Verification items for the finished model (mm, model axes). Face numbers are marked on the shaded views. A direction names the side the tool comes from. Give positions to 0.01 mm unless a question says otherwise; leave off trailing zeros. Loops run counter-clockwise (first coordinate to the right, second up) from the corner with the lowest first, then second, coordinate; pieces in that order, holes last. Notation, with made-up numbers: (-31, 25.25) - (22, 25.25) arc R23 ccw to (22, 51.25) - close; hole circle Ø10 at (55, -9.5). An arc over 180 degrees is marked (long way). One line per question, with ' | ' between items. Start each with the question number.
1. Depth check by flat-ended pin: pin 1 Ø10 at (x, z) = (83.5, -2) entering from +Y; pin 2 Ø16 at (x, y) = (82.5, 2.5) entering from -Z; pin 3 Ø10 at (x, y) = (85.5, 2.5) entering from +Z. Enter the tip coordinate at first touch or a pass-through.
2. Thickness scan on line 1 along X through (y, z) = (-10, 9); line 2 along X through (y, z) = (-11, 1); line 3 along Y through (x, z) = (58.5, 5.5). Record the ranges inside material, lowest first. Write a range as from..to.
3. Tool access check on the marked faces 1, 2, 3 and 4. Record the directions out of +Z, -Z, +X, -X, +Y, -Y that give a thin tool (end or side, any length) a straight path to the whole face; none if there is none.
4. Section check A-A, the plane z = -7.75. Enter the section's corners in (x, y), then the cut area to 3 significant figures.
5. Section check B-B, the plane x = 0. Enter the section's corners in (y, z).
6. Section check C-C, the plane z = 1. Enter the section's corners in (x, y).
7. Mould release check, pull along X, two halves, no side actions. Record for the marked faces 5 and 6: +X half, -X half, draft (parallel to the pull), parting line (faces both ways), or undercut.
8. Section check D-D, the plane y = -14. Enter the section's corners in (x, z), then the cut area to 3 significant figures.
Autodesk Fusion 360 part; units mm, degrees
sketch "Sketch1" plane through (0, 0, 0) normal (0, 0, 1) x (1, 0, 0)
  circle A0 centre (0, 0) radius 30
  circle A1 centre (129, 0) radius 20
  line L0 (0, 0) -> (0, 0)
  line L1 (0, 0) -> (0, 0)
  line L2 (0, 0) -> (0, 0)
  line L3 (0, 0) -> (0, 0)
  line L4 (0, 0) -> (0, 0)
  line L5 (0, 0) -> (0, 0)
  line L6 (-11.547, 20) -> (-23.094, 0)
  line L7 (-23.094, 0) -> (-11.547, -20)
  line L8 (-11.547, -20) -> (11.547, -20)
  line L9 (11.547, -20) -> (23.094, 0)
  line L10 (23.094, 0) -> (11.547, 20)
  line L11 (11.547, 20) -> (-11.547, 20)
  line L12 (129, 15) -> (114.7342, 4.6353)
  line L13 (114.7342, 4.6353) -> (120.1832, -12.1353)
  line L14 (120.1832, -12.1353) -> (137.8168, -12.1353)
  line L15 (137.8168, -12.1353) -> (143.2658, 4.6353)
  line L16 (143.2658, 4.6353) -> (129, 15)
  line L17 (0, 0) -> (129, 0) construction
  line L18 (28.2843, 10) -> (111.6795, 10)
  line L19 (28.2843, -10) -> (111.6795, -10)
  line L20 (40, 5) -> (100, 5)
  line L21 (40, -5) -> (100, -5)
  arc A2 (40, 5) -> (40, -5) centre (40, 0) ccw
  arc A3 (100, -5) -> (100, 5) centre (100, 0) ccw
  point P0 (129, 0)
  dimension "d1" = 60
  dimension "d2" = 129
  dimension "d3" = 40
  dimension "d4" = 20
  dimension "d5" = 15
extrude "Extrude1" add sketch "Sketch1" along normal mid plane 20 contours A0 | A1 makes body 1 at (25.0013, -16.5811, 3.3333) makes body 2 at (148.9006, -1.9914, -3.3333)
extrude "Extrude2" add sketch "Sketch1" along normal mid plane 12 contours A0 A1 L18 L19 bodies 1 2
sketch "Sketch3" plane through (0, 0, 0) normal (0, 0, 1) x (1, 0, 0)
sketch "Sketch4" plane through (0, 0, 0) normal (0, 0, 1) x (1, 0, 0)
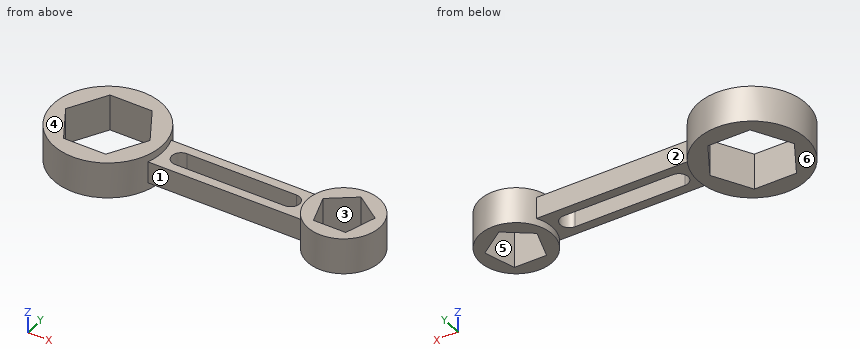
Results list:
1) pin 1: y = 10 | pin 2: z = -6 | pin 3: z = 6
2) line 1: -28.28..-17.32, 17.32..28.28, 111.68..119.49, 138.51..146.32 | line 2: -27.91..-16.74, 16.74..27.91, 112.3..119.81, 138.19..145.7 | line 3: -10..-5, 5..10
3) face 1: +Z, -Z, -Y | face 2: +Z, -Z, +Y | face 3: +Z, -Z | face 4: +Z, +X, -X, +Y, -Y
4) outline: circle Ø60 at (0, 0); circle Ø40 at (129, 0); hole (-23.09, 0) - (-11.55, -20) - (11.55, -20) - (23.09, 0) - (11.55, 20) - (-11.55, 20) - close; hole (114.73, 4.64) - (120.18, -12.14) - (137.82, -12.14) - (143.27, 4.64) - (129, 15) - close | area: 2,160 mm²
5) outline: (-30, -10) - (-20, -10) - (-20, 10) - (-30, 10) - close; (20, -10) - (30, -10) - (30, 10) - (20, 10) - close
6) outline: (28.28, -10) - (111.68, -10) arc R20 ccw (long way) to (111.68, 10) - (28.28, 10) arc R30 ccw (long way) to start; hole (-23.09, 0) - (-11.55, -20) - (11.55, -20) - (23.09, 0) - (11.55, 20) - (-11.55, 20) - close; hole (40, -5) - (100, -5) arc R5 ccw to (100, 5) - (40, 5) arc R5 ccw to start; hole (114.73, 4.64) - (120.18, -12.14) - (137.82, -12.14) - (143.27, 4.64) - (129, 15) - close
7) face 5: undercut | face 6: draft
8) outline: (-26.53, -10) - (-15.01, -10) - (-15.01, 10) - (-26.53, 10) - close; (15.01, -10) - (26.53, -10) - (26.53, 10) - (15.01, 10) - close; (114.72, -10) - (143.28, -10) - (143.28, 10) - (114.72, 10) - close | area: 1,030 mm²
